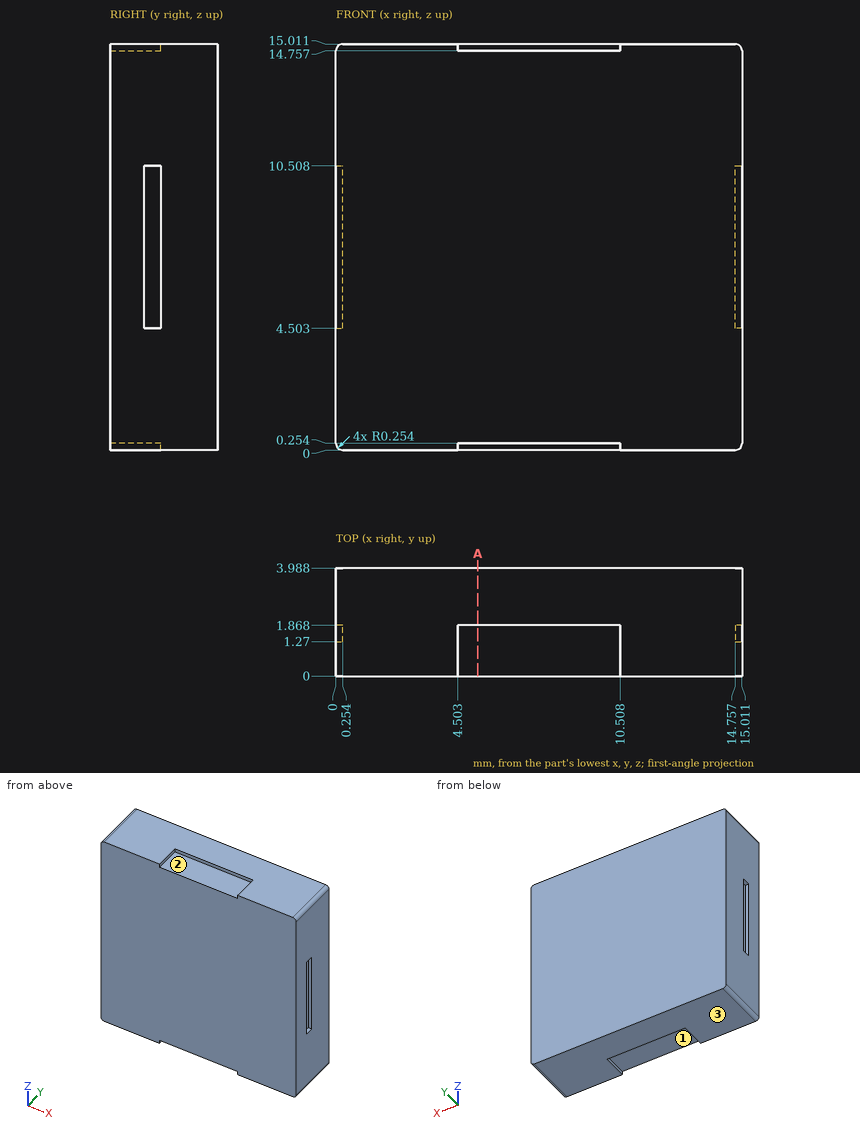
Input: dimensioned drawing with shaded views. Units: mm. Origin: part minimum x, y, z. A direction names the side the tool comes from. Give positions to 0.01 mm unless a question says otherwise; leave off trailing zeros. Write each loop counter-clockwise with the first axis right and the second up, starting at its lowest first coordinate (ties: lowest second). Pieces come first, ordered by that corner, then holes.
1. Reachability of the marked faces 1, 2 and 3 from +Z, -Z, +X, -X, +Y, -Y: full face, straight path, thin tool, end or side. Return the list, or none.
2. Section query A-A, the plane x = 5.25. Return loops of the section in (y, z).
3. Line query: probe 1 along Z at (x, y) = (9.75, 0.95). Output: solid intervals per line, ascending.
Computed:
1. face 1: -Z, -Y
1. face 2: +Z, -Y
1. face 3: -Z, +X, -X, +Y, -Y
2. outline: (0, 0.25) - (1.87, 0.25) - (1.87, 0) - (3.99, 0) - (3.99, 15.01) - (1.87, 15.01) - (1.87, 14.76) - (0, 14.76) - close
3. probe 1: z = 0.25 to 14.76
